Can you work these out from the model? Positions are in its coordinate system, mm. A direction names the side the tool comes from. Give positions to 0.01 mm unless a question says otherwise; leave off trailing zeros. Order: outer loops, then holes, each group sorted by start corner. A loop starts at its lowest first (then second) coordinate and runs counter-clockwise, first axis right, second up. Notation, with made-up numbers: (13, 89.25) - (57, 89.25) arc R11 cw to (57, 94.25) - close; hole circle Ø10 at (18.25, 69.25). An arc over 180 degrees is marked (long way). Answer as a JSON object with one key per item and string values.
```python
from build123d import *

# Parameters (mm, degrees)
F0_W     = 550
F0_H     = 550
F0_R     = 12.05
F1_DEPTH = 20
F2_R     = 5
F3_R     = 200
F4_DEPTH = 5


with BuildPart() as f1:
    # F0 (on Top) → F1 (new body)
    with BuildSketch(Plane.XY):
        Rectangle(F0_W, F0_H)
        Circle(F0_R, mode=Mode.SUBTRACT)
    extrude(amount=F1_DEPTH)

    # F2
    f2_edges = [f1.edges().sort_by_distance(p)[0] for p in [
        (-275, -275, 10),
        (275, -275, 10),
        (275, 275, 10),
        (-275, 275, 10),
    ]]
    fillet(f2_edges, radius=F2_R)

    # F3 (on face) → F4 (cut)
    with BuildSketch(Plane.XY.offset(20)):
        Circle(F3_R)
    extrude(amount=-F4_DEPTH, mode=Mode.SUBTRACT)


solid = f1.part
```
Q1. I need wall thicknesses on L1, parallel to X at y = 0, z = 11.25; L2, parallel to Y at x = 0, z = 17. Which ranges of each line are inside material? Lowest first, please.
Recorded:
{"L1": "x = -275 to -12.05, 12.05 to 275", "L2": "y = -275 to -200, 200 to 275"}
Q2. If we section it at A-A, the plane y = 0: Please give me the cut outline in (x, z), then the cut area to 3 significant figures.
Recorded:
{"outline": "(-275, 0) - (-12.05, 0) - (-12.05, 15) - (-200, 15) - (-200, 20) - (-275, 20) - close; (12.05, 0) - (275, 0) - (275, 20) - (200, 20) - (200, 15) - (12.05, 15) - close", "area": "8,640 mm^2"}
Q3. If we section it at D-D, the plane x = -75.5: Please give me the cut outline in (y, z).
Recorded:
{"outline": "(-275, 0) - (275, 0) - (275, 20) - (185.2, 20) - (185.2, 15) - (-185.2, 15) - (-185.2, 20) - (-275, 20) - close"}
Q4. Which directions (+Z, -Z, +X, -X, +Y, -Y) give clear straight access to the entire face, cutting with the end or side of a thin tool? Please do faces 1 (the face through (190.764, 60.075, 17.535)), 2 (the face through (-4, 275, 10)).
Recorded:
{"face 1": "+Z", "face 2": "+Z, -Z, +X, -X, +Y"}
Q5. If we section it at C-C, the plane y = 178: Please give me the cut outline in (x, z), then the cut area to 3 significant figures.
Recorded:
{"outline": "(-275, 0) - (275, 0) - (275, 20) - (91.19, 20) - (91.19, 15) - (-91.19, 15) - (-91.19, 20) - (-275, 20) - close", "area": "10,100 mm^2"}
Q6. We'd pull the mould along Y, two halves only. Please class faces 3 (the face through (-4, -275, 10)), 4 (the face through (-3, -42, 15)), 5 (the face through (275, -4, 10)): released by +Y, released by -Y, zero draft, split by the parting line, or undercut.
Recorded:
{"face 3": "released by -Y", "face 4": "undercut", "face 5": "zero draft"}
